For this review, use the dimensioned drawing (mm, ordinates from the lowest corner) and the shaded views. Round coordinates to 2 decimals unless told otherwise and drop trailing zeros. Write each loop counter-clockwise with the first axis right and the second up, starting at its lowest first coordinate (ties: lowest second). Pieces come first, ordered by that corner, then holes.
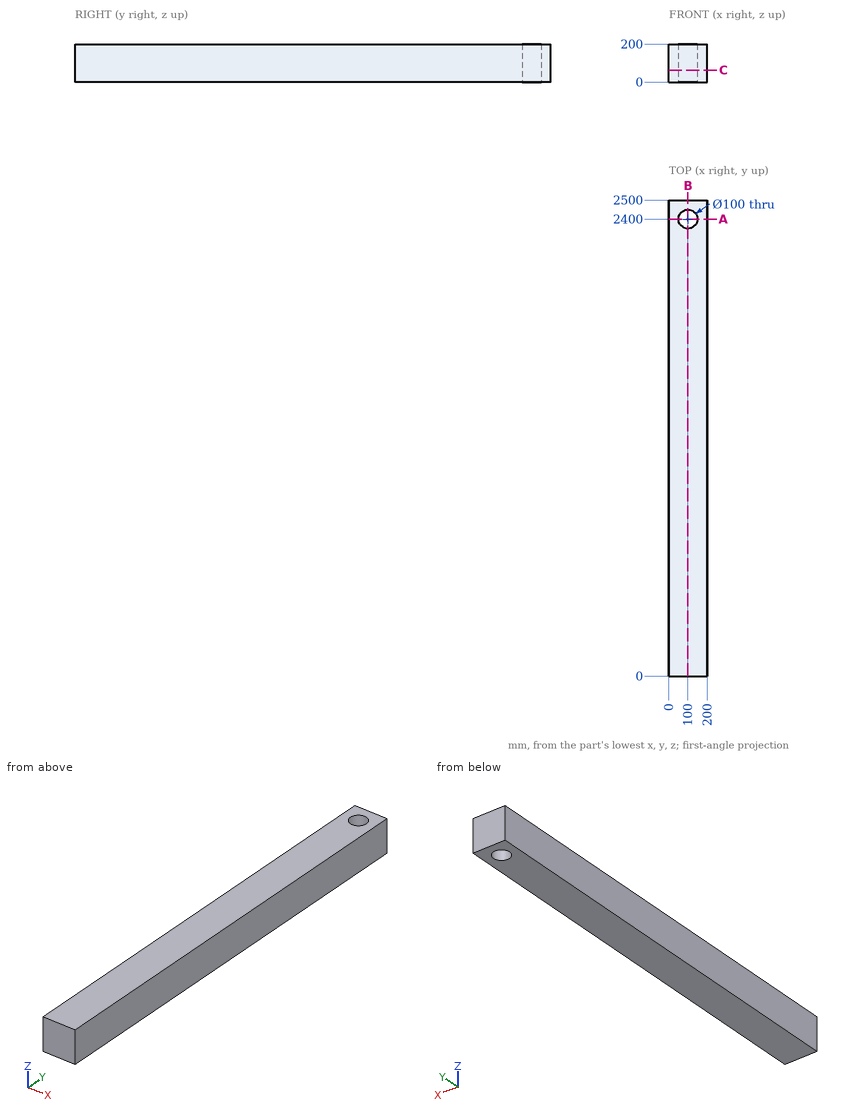
1) Add section A-A on y = 2400. State the section outline as (x, z) points.
2) Add section C-C on z = 63. State the section outline as (x, y) points.
3) Add section B-B on x = 100. State the section outline as (y, z) points, and give its area (3 significant figures).
4) For line 1 along Y through (x, z) = (100, 155); line 2 along Y through (x, z) = (97.5, 135.5); line 3 along X through (y, z) = (2400, 73), list the stretches that pass through material, from the lowest coordinate up.
Computed:
1. outline: (0, 0) - (50, 0) - (50, 200) - (0, 200) - close; (150, 0) - (200, 0) - (200, 200) - (150, 200) - close
2. outline: (0, 0) - (200, 0) - (200, 2500) - (0, 2500) - close; hole circle Ø100 at (100, 2400)
3. outline: (0, 0) - (2350, 0) - (2350, 200) - (0, 200) - close; (2450, 0) - (2500, 0) - (2500, 200) - (2450, 200) - close
3. area: 480,000 mm2
4. line 1: y = 0 to 2350, 2450 to 2500
4. line 2: y = 0 to 2350.06, 2449.94 to 2500
4. line 3: x = 0 to 50, 150 to 200
